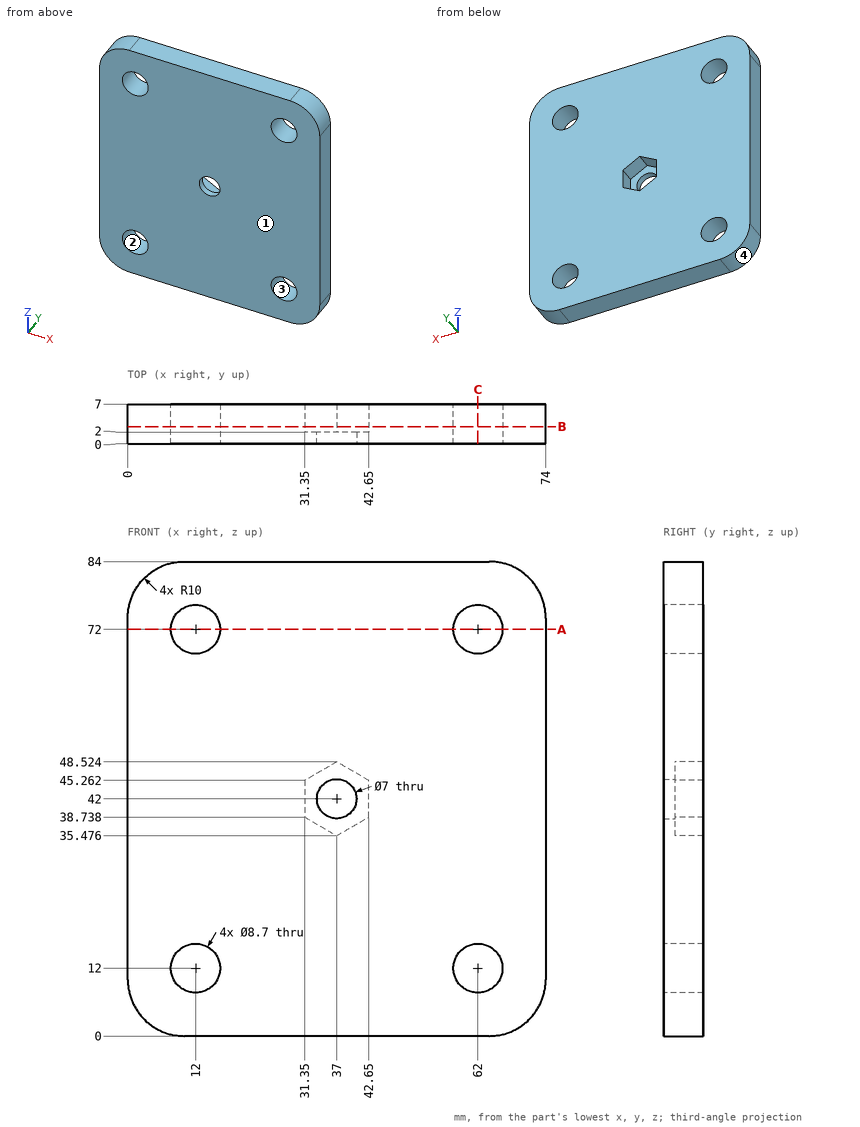
For this review, use the dimensioned drawing (mm, ordinates from the lowest corner) and the shaded views. Give positions to 0.01 mm unless a question says otherwise; leave off trailing zeros. Loops run counter-clockwise (first coordinate to the right, second up) from the corner with the lowest first, then second, coordinate; pieces in that order, holes last.
Item 1: Draft analysis for pull direction X (two halves, no side actions). For the marked faces 1, 2, 3 and 4, state which applies: +X half, -X half, draft (parallel to the pull), parting line (faces both ways), or undercut.
Item 2: Take a section at A-A, the plane z = 72. State the section outline as (x, y) points.
Item 3: Take a section at C-C, the plane x = 62. State the section outline as (y, z) points.
Item 4: Take a section at B-B, the plane y = 3. State the section outline as (x, z) points.
Item 5: For line 1 along Z through (x, y) = (12, 3); line 2 along X through (y, z) = (0.5, 42); line 3 along Z through (x, y) = (58, 1), list the stretches that pass through material, from the lowest coordinate up.
Calculated:
1. face 1: draft
1. face 2: undercut
1. face 3: undercut
1. face 4: -X half
2. outline: (0, 0) - (7.65, 0) - (7.65, 7) - (0, 7) - close; (16.35, 0) - (57.65, 0) - (57.65, 7) - (16.35, 7) - close; (66.35, 0) - (74, 0) - (74, 7) - (66.35, 7) - close
3. outline: (0, 0) - (7, 0) - (7, 7.65) - (0, 7.65) - close; (0, 16.35) - (7, 16.35) - (7, 67.65) - (0, 67.65) - close; (0, 76.35) - (7, 76.35) - (7, 84) - (0, 84) - close
4. outline: (0, 10) arc R10 ccw to (10, 0) - (64, 0) arc R10 ccw to (74, 10) - (74, 74) arc R10 ccw to (64, 84) - (10, 84) arc R10 ccw to (0, 74) - close; hole circle Ø8.7 at (12, 12); hole circle Ø8.7 at (12, 72); hole (31.35, 38.74) - (37, 35.48) - (42.65, 38.74) - (42.65, 45.26) - (37, 48.52) - (31.35, 45.26) - close; hole circle Ø8.7 at (62, 12); hole circle Ø8.7 at (62, 72)
5. line 1: z = 0 to 7.65, 16.35 to 67.65, 76.35 to 84
5. line 2: x = 0 to 33.5, 40.5 to 74
5. line 3: z = 0 to 10.29, 13.71 to 70.29, 73.71 to 84
